Verification items for the finished model (mm, model axes). A direction names the side the tool comes from. Coordinates: 2 decimals unless noted, no trailing zeros. Loops run counter-clockwise (first coordinate to the right, second up) from the corner with the lowest first, then second, coordinate; pieces in that order, holes last. Notation, with made-up numbers: (61, 1) - (66, 1) arc R30 ccw to (66, 24) - close; hole circle Ø7 at (72.25, -22.75). An arc over 180 degrees is marked (long way). Answer as CSV lines item,"result". Start each with the question number.
1. Set-up check for faces 5 (the flat face through (36, 16, 2)), 6 (the flat face through (15, 95, 2)), 7 (the flat face through (28, 130, 2)): record each of +Z, -Z, +X, -X, +Y, -Y from which the full face is reachable in a straight line by a thin tool's end or side.
2. Cross-section at A-A (x = 7.5). Enter the section's corners in (y, z).
3. Cross-section at C-C (x = 36). Enter the section's corners in (y, z).
4. Release check for a two-part mould opening along X. For faces 1 (the flat face through (42, 8, 2)), 2 (the cylindrical face through (37.478, 8.466, 2.465)), 3 (the flat face through (0, 30, 2)), 4 (the flat face through (36, 114, 2)) record: pulls with the +X half, pulls with the -X half, needs draft (parallel to the pull), parting line crosses it, or undercut.
5. Cross-section at B-B (y = 8). Enter the section's corners in (x, z), plus the area to 4 significant figures.
6. Cross-section at D-D (y = 122). Enter the section's corners in (x, z).
7. Material ranges on line 1 (X direction, y = 122, z = 3.6); line 2 (Y direction, x = 36, z = 3.6); line 3 (Y direction, x = 7.5, z = 2.35), recorded low to high. Write a range as [from, to].
8. Gauge pin test, flat ends, axial feed: P1, Ø1.5, axis at y = 79, z = 2, coming from the -X side; P2, Ø1.5, axis at x = 6, z = 3, coming from the +Y side. Record the tip position at first contact, or that the pin passes through.
```python
from build123d import *

# Parameters (mm, degrees)
SKETCH1_W           = 15
SKETCH1_H           = 60
SKETCH1_R           = 1.55
SKETCH1_W_2         = 12
SKETCH1_H_2         = 16
BOSS_EXTRUDE1_DEPTH = 5


with BuildPart() as part:
    # Sketch1 → Boss-Extrude1 (new body)
    # profile 1 of 4: a face of its own
    with BuildSketch(Plane.XY):
        with Locations((7.5, 30)):
            Rectangle(SKETCH1_W, SKETCH1_H)
        with Locations((7.5, 8)):
            Circle(SKETCH1_R, mode=Mode.SUBTRACT)
        with Locations((7.5, 52)):
            Circle(SKETCH1_R, mode=Mode.SUBTRACT)
    # profile 2 of 4: a face of its own
    with BuildSketch(Plane.XY):
        Polygon((15, 60), (15, 0), (30, 0), (30, 16), (30, 114), (30, 130), (15, 130), align=None)
        with Locations((22.5, 8)):
            Circle(SKETCH1_R, mode=Mode.SUBTRACT)
        with Locations((22.5, 122)):
            Circle(SKETCH1_R, mode=Mode.SUBTRACT)
    # profile 3 of 4: a face of its own
    with BuildSketch(Plane.XY):
        with Locations((36, 8)):
            Rectangle(SKETCH1_W_2, SKETCH1_H_2)
        with Locations((36, 8)):
            Circle(SKETCH1_R, mode=Mode.SUBTRACT)
    # profile 4 of 4: a face of its own
    with BuildSketch(Plane.XY):
        with Locations((36, 122)):
            Rectangle(SKETCH1_W_2, SKETCH1_H_2)
        with Locations((36, 122)):
            Circle(SKETCH1_R, mode=Mode.SUBTRACT)
    extrude(amount=BOSS_EXTRUDE1_DEPTH)


solid = part.part
```
Values follow:
1,face 5,"+Z, -Z, +X"
1,face 6,"+Z, -Z, -X, +Y"
1,face 7,"+Z, -Z, +X, -X, +Y"
2,outline,"(0, 0) - (6.45, 0) - (6.45, 5) - (0, 5) - close; (9.55, 0) - (50.45, 0) - (50.45, 5) - (9.55, 5) - close; (53.55, 0) - (60, 0) - (60, 5) - (53.55, 5) - close"
3,outline,"(0, 0) - (6.45, 0) - (6.45, 5) - (0, 5) - close; (9.55, 0) - (16, 0) - (16, 5) - (9.55, 5) - close; (114, 0) - (120.45, 0) - (120.45, 5) - (114, 5) - close; (123.55, 0) - (130, 0) - (130, 5) - (123.55, 5) - close"
4,face 1,"pulls with the +X half"
4,face 2,"undercut"
4,face 3,"pulls with the -X half"
4,face 4,"needs draft"
5,outline,"(0, 0) - (5.95, 0) - (5.95, 5) - (0, 5) - close; (9.05, 0) - (20.95, 0) - (20.95, 5) - (9.05, 5) - close; (24.05, 0) - (34.45, 0) - (34.45, 5) - (24.05, 5) - close; (37.55, 0) - (42, 0) - (42, 5) - (37.55, 5) - close"
5,area,"163.5 mm²"
6,outline,"(15, 0) - (20.95, 0) - (20.95, 5) - (15, 5) - close; (24.05, 0) - (34.45, 0) - (34.45, 5) - (24.05, 5) - close; (37.55, 0) - (42, 0) - (42, 5) - (37.55, 5) - close"
7,line 1,"x = [15, 20.95], [24.05, 34.45], [37.55, 42]"
7,line 2,"y = [0, 6.45], [9.55, 16], [114, 120.45], [123.55, 130]"
7,line 3,"y = [0, 6.45], [9.55, 50.45], [53.55, 60]"
8,P1,"stops at x = 15"
8,P2,"stops at y = 60"
